```python
from build123d import *

# Parameters (mm, degrees)
SKETCH_1_R                  = 2
SKETCH_1_R_2                = 1.7
SKETCH_1_W                  = 6.6
SKETCH_1_H                  = 30
F_09_C920_TRIPOD_TRAY_DEPTH = 5


with BuildPart() as part:
    # Эскиз1 → 09_C920_tripod_tray (new body)
    with BuildSketch(Plane.XY):
        Polygon((-51, -42.5), (51, -42.5), (63, -30.5), (63, 30.5), (51, 42.5), (-51, 42.5), (-63, 30.5), (-63, -30.5), align=None)
        with Locations((-53, -26)):
            Circle(SKETCH_1_R, mode=Mode.SUBTRACT)
        with Locations((-53, 26)):
            Circle(SKETCH_1_R, mode=Mode.SUBTRACT)
        with Locations((53, -26)):
            Circle(SKETCH_1_R_2, mode=Mode.SUBTRACT)
        with Locations((53, 26)):
            Circle(SKETCH_1_R_2, mode=Mode.SUBTRACT)
        Rectangle(SKETCH_1_W, SKETCH_1_H, mode=Mode.SUBTRACT)
    extrude(amount=F_09_C920_TRIPOD_TRAY_DEPTH)


solid = part.part
```
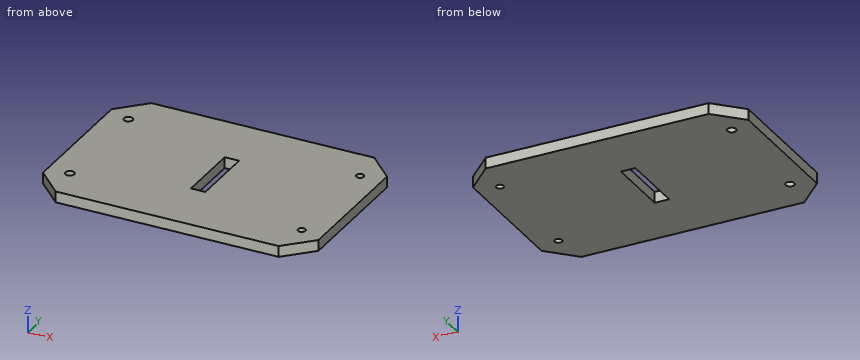
Input: part model. Units: mm. Frame: model coordinates. Give positions to 0.01 mm unless a question says otherwise; leave off trailing zeros. Order: outer loops, then holes, each group sorted by start corner. A loop starts at its lowest first (then second) coordinate and runs counter-clockwise, first axis right, second up. Notation, with made-up numbers: (28, 83) - (81, 83) arc R26 ccw to (81, 105) - close; hole circle Ø10 at (31, 64.25). An arc over 180 degrees is marked (long way). Put each result on its own line as item: value.
Item 1: Section query D-D, the plane y = 2. Return loops of the section in (x, z), then the cut area to 3 significant figures.
Found:
outline: (-63, 0) - (-3.3, 0) - (-3.3, 5) - (-63, 5) - close; (3.3, 0) - (63, 0) - (63, 5) - (3.3, 5) - close
area: 597 mm^2
Item 2: Section query B-B, the plane x = -53. Return loops of the section in (y, z), then the cut area to 3 significant figures.
Found:
outline: (-40.5, 0) - (-28, 0) - (-28, 5) - (-40.5, 5) - close; (-24, 0) - (24, 0) - (24, 5) - (-24, 5) - close; (28, 0) - (40.5, 0) - (40.5, 5) - (28, 5) - close
area: 365 mm^2
Item 3: Section query C-C, the plane z = 0.75. Return loops of the section in (x, y), then the cut area to 3 significant figures.
Found:
outline: (-63, -30.5) - (-51, -42.5) - (51, -42.5) - (63, -30.5) - (63, 30.5) - (51, 42.5) - (-51, 42.5) - (-63, 30.5) - close; hole circle Ø4 at (-53, -26); hole circle Ø4 at (-53, 26); hole (-3.3, -15) - (3.3, -15) - (3.3, 15) - (-3.3, 15) - close; hole circle Ø3.4 at (53, -26); hole circle Ø3.4 at (53, 26)
area: 10,200 mm^2
Item 4: Ray query, L1, parallel to X at y = 1, z = 0.4; L2, parallel to Y at x = 52, z = 3.05; L3, parallel to Y at x = 53, z = 2.1. Return the intervals inside material, ascending. Write a range as from..to.
Found:
L1: x = -63..-3.3, 3.3..63
L2: y = -41.5..-27.37, -24.63..24.63, 27.37..41.5
L3: y = -40.5..-27.7, -24.3..24.3, 27.7..40.5
Item 5: Section query A-A, the plane y = 26. Return loops of the section in (x, z).
Found:
outline: (-63, 0) - (-55, 0) - (-55, 5) - (-63, 5) - close; (-51, 0) - (51.3, 0) - (51.3, 5) - (-51, 5) - close; (54.7, 0) - (63, 0) - (63, 5) - (54.7, 5) - close
Item 6: Contact query for flat-ended pins moving along their axis: pin 1 (2 mm diameter, centred on x = 53, y = -26, fed in from -Z) (3 decimals); pin 2 (4.5 mm diameter, centred on x = -53, y = -26, fed in from +Z). Output: stop coordinate, or through.
Found:
pin 1: passes through
pin 2: stops at z = 5
